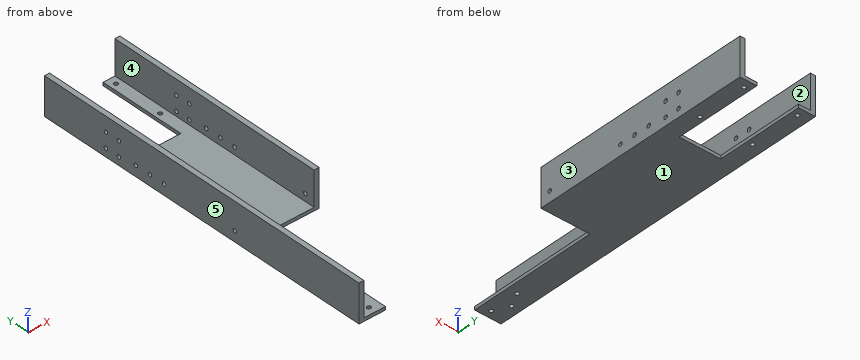
from build123d import *

# Parameters (mm, degrees)
BOSS_EXTRUDE1_DEPTH     = 177.8
SKETCH2_R               = 2
SKETCH2_W               = 21.020738686
SKETCH2_H               = 87.907641246
CUT_EXTRUDE1_DEPTH      = 4.302
SKETCH4_R               = 2
CUT_EXTRUDE2_DEPTH      = 4.302
SKETCH5_R               = 2
CUT_EXTRUDE3_DEPTH      = 77.2
CUT_EXTRUDE4_DEPTH      = 1
CUT_EXTRUDE4_DEPTH_BACK = 39.1


with BuildPart() as part:
    # Sketch1 → Boss-Extrude1 (new body, symmetric)
    with BuildSketch(Plane(origin=(0, 0, 0), x_dir=(1, 0, 0), z_dir=(0, 1, 0))):
        Polygon((-38.1, -19.05), (-33.02, -19.05), (-33.02, 15.748), (33.02, 15.748), (33.02, -19.05), (38.1, -19.05), (38.1, 19.05), (-38.1, 19.05), align=None)
    extrude(amount=BOSS_EXTRUDE1_DEPTH, both=True)

    # Sketch2 → Cut-Extrude1 (cut, through all)
    with BuildSketch(Plane.XY.offset(-15.748)):
        with Locations((-27.020369343, 169.8)):
            Circle(SKETCH2_R)
        with Locations((-26.52, 119.475689004)):
            Circle(SKETCH2_R)
        with Locations((-10.510369343, 133.846179377)):
            Rectangle(SKETCH2_W, SKETCH2_H)
    cut_extrude1 = extrude(amount=-CUT_EXTRUDE1_DEPTH, mode=Mode.SUBTRACT)

    # Mirror1: Cut-Extrude1 across plane
    add(cut_extrude1.mirror(Plane(origin=(0, 0, 0), x_dir=(0, 0, 1), z_dir=(1, 0, 0))), mode=Mode.SUBTRACT)

    # Sketch4 → Cut-Extrude2 (cut, through all)
    with BuildSketch(Plane.XY.offset(-15.748)):
        with Locations((-21.335, -170.3)):
            Circle(SKETCH4_R)
        with Locations((-28.835, -155.575)):
            Circle(SKETCH4_R)
        with Locations((-21.335, -140.85)):
            Circle(SKETCH4_R)
    extrude(amount=-CUT_EXTRUDE2_DEPTH, mode=Mode.SUBTRACT)

    # Sketch5 → Cut-Extrude3 (cut, through all)
    with BuildSketch(Plane.ZY.offset(38.1)):
        with Locations((-8.375, 58.5851)):
            Circle(SKETCH5_R)
        with Locations((-8.375, 74.5851)):
            Circle(SKETCH5_R)
        with Locations((-8.375, 42.5851)):
            Circle(SKETCH5_R)
        with Locations((-8.375, -37.4269)):
            Circle(SKETCH5_R)
        with Locations((-10.875, 93.638)):
            Circle(SKETCH5_R)
        with Locations((4.125, 93.638)):
            Circle(SKETCH5_R)
        with Locations((4.125, 108.363)):
            Circle(SKETCH5_R)
        with Locations((-10.875, 108.363)):
            Circle(SKETCH5_R)
    extrude(amount=-CUT_EXTRUDE3_DEPTH, mode=Mode.SUBTRACT)

    # Sketch6 → Cut-Extrude4 (cut, two sides)
    with BuildSketch(Plane.XY.offset(19.05)) as cut_extrude4_sk:
        Polygon((766.139495362, -47.4269), (38.1, -47.4269), (-11.335, -47.4269), (-11.335, -177.8), (-11.335, -905.839495362), (1067.889453991, -1883.30591685), (1845.363949353, -1024.893321488), align=None)
    extrude(amount=CUT_EXTRUDE4_DEPTH, mode=Mode.SUBTRACT)
    extrude(cut_extrude4_sk.sketch, amount=-CUT_EXTRUDE4_DEPTH_BACK, mode=Mode.SUBTRACT)


solid = part.part
Check sheet for the modelled part. Datum: model origin and axes. Units: mm. Face numbers are marked on the shaded views. A direction names the side the tool comes from. Coordinates: 2 decimals unless noted, no trailing zeros. Loops run counter-clockwise (first coordinate to the right, second up) from the corner with the lowest first, then second, coordinate; pieces in that order, holes last. Notation, with made-up numbers: (-28, -12.75) -> (-8, -12.75) arc R21 ccw to (-8, 22.25) -> close; hole circle Ø4 at (59, -0.5). An arc over 180 degrees is marked (long way). Answer in a Markdown table with one row per item.
1. Access from +Z, -Z, +X, -X, +Y, -Y to the whole of each face (thin tool, end or side, straight path). Record for the marked faces 4 and 5.
Check values:
| item | result |
|---|---|
| face 4 | +Z, +Y, -Y |
| face 5 | +Z, -Z, -X, +Y, -Y |
2. Sectioned sample at D-D, the plane y = -68. Record the boundary of the cut face in (x, z) (3 decimals).
Check values:
| item | result |
|---|---|
| outline | (-38.1, -19.05) -> (-11.335, -19.05) -> (-11.335, -15.748) -> (-33.02, -15.748) -> (-33.02, 19.05) -> (-38.1, 19.05) -> close |
3. Go/stop test with flat-tipped pins: pin 1 (2.5 mm diameter, centred on x = -28.835, y = -155.575, fed in from -Z); pin 2 (6.5 mm diameter, centred on x = 26.52, y = 119.48, fed in from -Z); pin 3 (1.7 mm diameter, centred on x = -4.5, z = -16.5, fed in from +Y); pin 4 (6 mm diameter, centred on x = -22.5, y = 132, fed in from +Z). Record where each tip stops, or that it passes through.
Check values:
| item | result |
|---|---|
| pin 1 | passes through |
| pin 2 | stops at z = -19.05 |
| pin 3 | stops at y = 89.89 |
| pin 4 | stops at z = -15.75 |
4. Sectioned sample at B-B, the plane y = -26. Record the boundary of the cut face in (x, z).
Check values:
| item | result |
|---|---|
| outline | (-38.1, -19.05) -> (38.1, -19.05) -> (38.1, 19.05) -> (33.02, 19.05) -> (33.02, -15.75) -> (-33.02, -15.75) -> (-33.02, 19.05) -> (-38.1, 19.05) -> close |
5. Sectioned sample at C-C, the plane x = -7.5. Record the boundary of the cut face in (y, z).
Check values:
| item | result |
|---|---|
| outline | (-47.43, -19.05) -> (89.89, -19.05) -> (89.89, -15.75) -> (-47.43, -15.75) -> close |
6. Sectioned sample at A-A, the plane z = 11.5. Record the boundary of the cut face in (x, y).
Check values:
| item | result |
|---|---|
| outline | (-38.1, -177.8) -> (-33.02, -177.8) -> (-33.02, 177.8) -> (-38.1, 177.8) -> close; (33.02, -47.43) -> (38.1, -47.43) -> (38.1, 177.8) -> (33.02, 177.8) -> close |
7. Material ranges on line 1 along X through (y, z) = (-170.3, -17.6) (3 decimals); line 2 along X through (y, z) = (100, -3.5); line 3 along Z through (x, y) = (-22.5, -101), recorded low to high. Write a range as [from, to].
Check values:
| item | result |
|---|---|
| line 1 | x = [-38.1, -23.335], [-19.335, -11.335] |
| line 2 | x = [-38.1, -33.02], [33.02, 38.1] |
| line 3 | z = [-19.05, -15.75] |
8. Release check for a two-part mould opening along X. For the marked faces 1, 2 and 3 record: released by +X, released by -X, zero draft, split by the parting line, or undercut.
Check values:
| item | result |
|---|---|
| face 1 | zero draft |
| face 2 | undercut |
| face 3 | released by +X |
